Answer from the drawing. Dimensions are ordinates in mm from the lowest x, y and z of the part. A direction names the side the tool comes from. Coordinates: 2 decimals unless noted, no trailing zeros. Order: outer loops, then holes, each group sorted by start corner. A loop starts at its lowest first (then second) coordinate and runs counter-clockwise, first axis right, second up. Notation, with made-up numbers: (-38, 18.25) -> (16, 18.25) arc R19 ccw to (16, 25.25) -> close; hole circle Ø10 at (73, 51.25). An arc over 180 degrees is marked (long way). Answer in a Markdown table with one row per item.
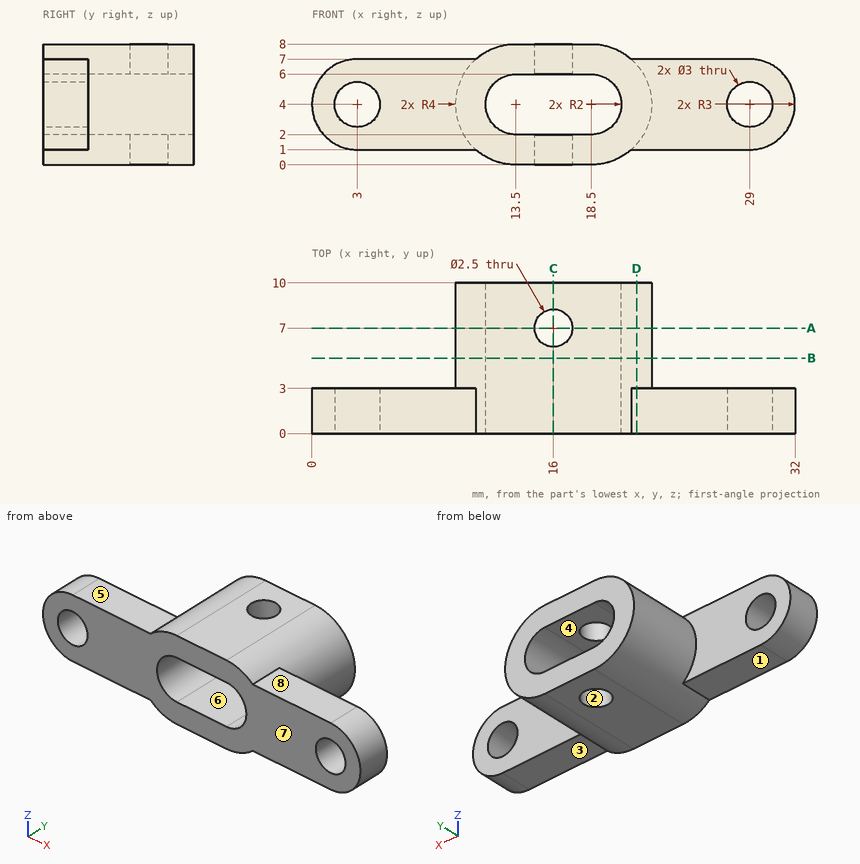
(1) A cutting plane is placed at C-C, the plane x = 16. Determine the outline of the cut face in (y, z).
Check values:
| item | result |
|---|---|
| outline | (0, 0) -> (5.75, 0) -> (5.75, 2) -> (0, 2) -> close; (0, 6) -> (5.75, 6) -> (5.75, 8) -> (0, 8) -> close; (8.25, 0) -> (10, 0) -> (10, 2) -> (8.25, 2) -> close; (8.25, 6) -> (10, 6) -> (10, 8) -> (8.25, 8) -> close |
(2) Which of the six approach directions +Z, -Z, +X, -X, +Y, -Y give full straight-line access (tool end or side, diameter ignored) to the marked faces 1, 2, 3, 4 and 5?
Check values:
| item | result |
|---|---|
| face 1 | -Z, -X, +Y, -Y |
| face 2 | +Z, -Z |
| face 3 | -Z, +X, +Y, -Y |
| face 4 | +Y, -Y |
| face 5 | +Z, -X, +Y, -Y |
(3) Flat-ended cylindrical pins translate along their axes: pin 1 (5 mm diameter, centred on x = 21.5, y = 7, fed in from -Z); pin 2 (1.5 mm diameter, centred on x = 7.5, y = 2, fed in from +Z); pin 3 (3 mm diameter, centred on x = 7.5, z = 3, fed in from +Y); pin 4 (1.5 mm diameter, centred on x = 16, y = 7, fed in from +Z). Find the tip coordinate at first contact, or state that the pin passes through.
Check values:
| item | result |
|---|---|
| pin 1 | z = 0.03 |
| pin 2 | z = 7 |
| pin 3 | y = 3 |
| pin 4 | through |
(4) Find the intervals of material crossed by line 1 along Y through (x, z) = (16, 6.7); line 2 along Y through (x, z) = (6, 3.25); line 3 along Z through (x, y) = (18, 7.5), in increasing order. Write a range as from..to.
Check values:
| item | result |
|---|---|
| line 1 | 0..5.75, 8.25..10 |
| line 2 | 0..3 |
| line 3 | 0..2, 6..8 |
(5) A cutting plane is placed at B-B, the plane y = 5. Determine the outline of the cut face in (x, z), then the cut area to 3 significant figures.
Check values:
| item | result |
|---|---|
| outline | (13.5, 0) -> (18.5, 0) arc R4 ccw to (18.5, 8) -> (13.5, 8) arc R4 ccw to start; hole (13.5, 2) -> (18.5, 2) arc R2 ccw to (18.5, 6) -> (13.5, 6) arc R2 ccw to start |
| area | 57.7 mm² |
(6) A cutting plane is placed at D-D, the plane x = 21.5. Determine the outline of the cut face in (y, z), then the cut area to 3 significant figures.
Check values:
| item | result |
|---|---|
| outline | (0, 1) -> (3, 1) -> (3, 1.35) -> (10, 1.35) -> (10, 6.65) -> (3, 6.65) -> (3, 7) -> (0, 7) -> close |
| area | 55.0 mm² |
(7) A cutting plane is placed at A-A, the plane y = 7. Determine the outline of the cut face in (x, z).
Check values:
| item | result |
|---|---|
| outline | (13.5, 0) -> (14.75, 0) -> (14.75, 2) -> (13.5, 2) arc R2 cw to (13.5, 6) -> (14.75, 6) -> (14.75, 8) -> (13.5, 8) arc R4 ccw to start; (17.25, 0) -> (18.5, 0) arc R4 ccw to (18.5, 8) -> (17.25, 8) -> (17.25, 6) -> (18.5, 6) arc R2 cw to (18.5, 2) -> (17.25, 2) -> close |
(8) For a pull along Z with two mould halves and no side action, classify the marked faces 6, 7 and 8 as released by +Z, released by -Z, zero draft, split by the parting line, or undercut.
Check values:
| item | result |
|---|---|
| face 6 | undercut |
| face 7 | zero draft |
| face 8 | released by +Z |
